```python
from build123d import *

# Parameters (mm, degrees)
SCHIZZO1_R                   = 1
ESTRUSIONE_ESTRUSIONE1_DEPTH = 20
SCHIZZO2_R                   = 2.05
ESTRUSIONE_ESTRUSIONE2_DEPTH = 1.2
RACCORDO1_R                  = 0.5
TAGLIO_ESTRUSIONE1_DEPTH     = 0.5


with BuildPart() as part:
    # Schizzo1 → Estrusione-Estrusione1 (new body)
    with BuildSketch(Plane.XY):
        Circle(SCHIZZO1_R)
    extrude(amount=ESTRUSIONE_ESTRUSIONE1_DEPTH)

    # Schizzo2 → Estrusione-Estrusione2 (add)
    with BuildSketch(Plane(origin=(0, 0, 0), x_dir=(-1, 0, 0), z_dir=(0, 0, -1))):
        Circle(SCHIZZO2_R)
    extrude(amount=ESTRUSIONE_ESTRUSIONE2_DEPTH)

    # Raccordo1
    raccordo1_edges = [part.edges().sort_by_distance(p)[0] for p in [
        (2.05, 0, -1.2),
    ]]
    fillet(raccordo1_edges, radius=RACCORDO1_R)

    # Schizzo3 → Taglio-Estrusione1 (cut)
    with BuildSketch(Plane(origin=(0, 0, -1.2), x_dir=(-1, 0, 0), z_dir=(0, 0, -1))):
        Polygon((-0.25, 0.25), (-1, 0.25), (-1, -0.25), (-0.25, -0.25), (-0.25, -1), (0.25, -1), (0.25, -0.25), (1, -0.25), (1, 0.25), (0.25, 0.25), (0.25, 1), (-0.25, 1), align=None)
    extrude(amount=-TAGLIO_ESTRUSIONE1_DEPTH, mode=Mode.SUBTRACT)


solid = part.part
```
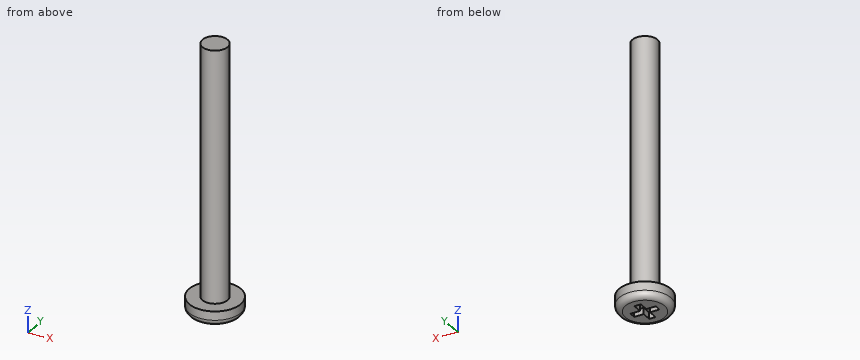
Input: part model. Units: mm. Frame: model coordinates. Round coordinates to 2 decimals unless told otherwise and drop trailing zeros. Order: outer loops, then holes, each group sorted by start corner. A loop starts at its lowest first (then second) coordinate and runs counter-clockwise, first axis right, second up. Notation, with made-up numbers: (82.25, 8) - (94.25, 8) arc R28 cw to (94.25, 40) - close; hole circle Ø11 at (14.25, 82). An arc over 180 degrees is marked (long way). One line per question, with ' | ' between items. Start each with the question number.
1) Cut plane A-A, the plane x = 0. Return the cut outline in (y, z), then the cut area to 3 significant figures.
2) Ray query, probe 1 along Z at (x, y) = (1, -0.4); probe 2 along X at (y, z) = (0.05, 12.5); probe 3 along Y at (x, z) = (0.55, 2.25). Return the intervals inside material, ascending.
3) Contact query for flat-ended pins moving along their axis: P1, Ø1, axis at x = 0.5, y = 0, coming from the -Z side; P2, Ø0.6, axis at y = -0.5, z = -1, coming from the +X side; P3, Ø1.5, axis at y = 1, z = 13.5, coming from the -X side; P4, Ø1.5, axis at x = 0.5, z = 1, coming from the -Y side. Output: stop coordinate, or through.
4) Cut plane C-C, the plane z = 6. Return the cut outline in (x, y), then the cut area to 3 significant figures.
Worked out:
1) outline: (-2.05, -0.7) arc R0.5 ccw to (-1.55, -1.2) - (-1, -1.2) - (-1, -0.7) - (1, -0.7) - (1, -1.2) - (1.55, -1.2) arc R0.5 ccw to (2.05, -0.7) - (2.05, 0) - (1, 0) - (1, 20) - (-1, 20) - (-1, 0) - (-2.05, 0) - close | area: 43.8 mm^2
2) probe 1: z = -1.2 to 0 | probe 2: x = -1 to 1 | probe 3: y = -0.84 to 0.84
3) P1: stops at z = -1.2 | P2: stops at x = 2.02 | P3: stops at x = -0.97 | P4: stops at y = -1
4) outline: circle Ø2 at (0, 0) | area: 3.14 mm^2
